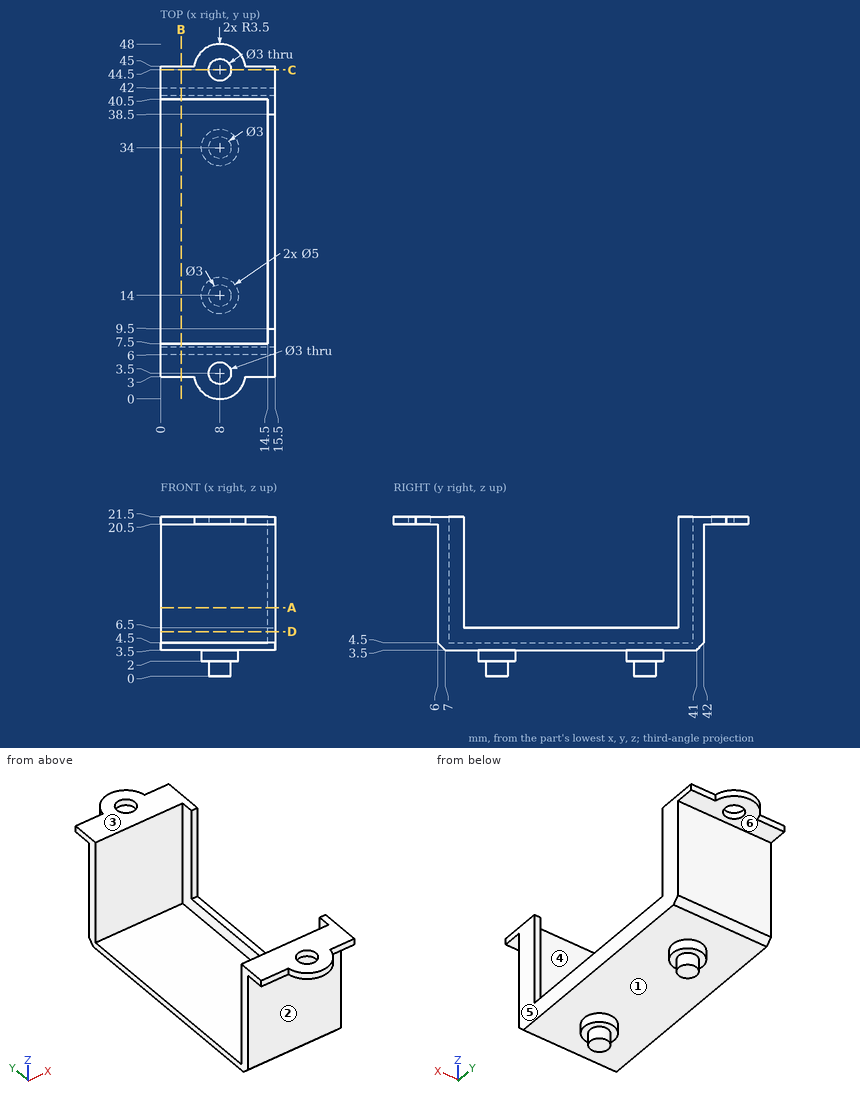
Input: dimensioned drawing with shaded views. Units: mm. Origin: part minimum x, y, z. A direction names the side the tool comes from. Coordinates: 2 decimals unless noted, no trailing zeros. Order: outer loops, then holes, each group sorted by start corner. A loop starts at its lowest first (then second) coordinate and runs counter-clockwise, first axis right, second up.
1. Access query for the marked faces 4, 5 and 6. Directions: +Z, -Z, +X, -X, +Y, -Y. A direction counts if a zero-diameter tool reaches every point of the face in a straight line with its end or side. Return the directions, or none.
Checked values:
face 4: +Z, -X
face 5: +Z, -Z, +X, +Y, -Y
face 6: -Z, +X, -X, +Y
2. Cut plane A-A, the plane z = 9.25. Return loops of the section in (x, y), plus the area to 3 significant figures.
Checked values:
outline: (0, 6) - (15.5, 6) - (15.5, 9.5) - (14.5, 9.5) - (14.5, 7.5) - (0, 7.5) - close; (0, 40.5) - (14.5, 40.5) - (14.5, 38.5) - (15.5, 38.5) - (15.5, 42) - (0, 42) - close
area: 50.5 mm2
3. Draft query along Y for the marked faces 1, 2 and 3. Return one class per face: +Y half, -Y half, draft (parallel to the pull), parting line (faces both ways), or undercut.
Checked values:
face 1: undercut
face 2: -Y half
face 3: draft
4. Cut plane B-B, the plane x = 2.75. Return loops of the section in (y, z), plus the area to 3 significant figures.
Checked values:
outline: (3, 20.5) - (6, 20.5) - (6, 4.5) - (7, 3.5) - (41, 3.5) - (42, 4.5) - (42, 20.5) - (45, 20.5) - (45, 21.5) - (40.5, 21.5) - (40.5, 4.5) - (7.5, 4.5) - (7.5, 21.5) - (3, 21.5) - close
area: 92.0 mm2
5. Cut plane D-D, the plane z = 6. Return loops of the section in (x, y).
Checked values:
outline: (0, 6) - (15.5, 6) - (15.5, 42) - (0, 42) - (0, 40.5) - (14.5, 40.5) - (14.5, 7.5) - (0, 7.5) - close
6. Contact query for flat-ended pins moving along their axis: P1, Ø4, axis at x = 6.5, z = 12, coming from the -Y side; P2, Ø1.1, axis at x = 13, z = 21, coming from the -Y side; P3, Ø2.5, axis at x = 8, y = 44.5, coming from the +Z side; P4, Ø0.8, axis at x = 15, z = 13.5, coming from the +Y side. Output: stop coordinate, or through.
Checked values:
P1: stops at y = 6
P2: stops at y = 3
P3: passes through
P4: stops at y = 42
7. Ray query, line 1 along Y through (x, z) = (8, 20.9); line 2 along Y through (x, z) = (4.5, 14.5); line 3 along X through (y, z) = (44.5, 21.05). Return the intervals inside material, ascending.
Checked values:
line 1: y = 0 to 2, 5 to 7.5, 40.5 to 43, 46 to 48
line 2: y = 6 to 7.5, 40.5 to 42
line 3: x = 0 to 6.5, 9.5 to 15.5
8. Cut plane C-C, the plane y = 44.5. Return loops of the section in (x, z).
Checked values:
outline: (0, 20.5) - (6.5, 20.5) - (6.5, 21.5) - (0, 21.5) - close; (9.5, 20.5) - (15.5, 20.5) - (15.5, 21.5) - (9.5, 21.5) - close
